Check sheet for the modelled part. Datum: model origin and axes. Units: mm. A direction names the side the tool comes from. Round coordinates to 2 decimals unless told otherwise and drop trailing zeros. Loops run counter-clockwise (first coordinate to the right, second up) from the corner with the lowest first, then second, coordinate; pieces in that order, holes last. Notation, with made-up numbers: (75, 52) -> (103, 52) arc R24 ccw to (103, 69) -> close; hole circle Ø10 at (29.25, 14.5). An arc over 180 degrees is marked (long way). Return JSON: item names as keys, results as strings.
from build123d import *

# Parameters (mm, degrees)
F0_W     = 76.597254
F0_H     = 76.218059
F1_DEPTH = 19.05
F2_R     = 25.573728
F3_DEPTH = 76.2
F4_W     = 76.946799
F4_H     = 75.848795
F5_DEPTH = 19.05
F8_D     = 12.7
F9_D     = 38.1


with BuildPart() as f1:
    # F0 (on Right) → F1 (new body)
    with BuildSketch(Plane.YZ):
        with Locations((-6.7307, 10.143448)):
            Rectangle(F0_W, F0_H)
    extrude(amount=F1_DEPTH)

    # F2 (on face) → F3 (join)
    with BuildSketch(Plane(origin=(0, 0, 0), x_dir=(0, -1, 0), z_dir=(-1, 0, 0))):
        with Locations((7.766344, 7.780468)):
            Circle(F2_R)
    extrude(amount=F3_DEPTH)

    # F4 (on face) → F5 (join)
    with BuildSketch(Plane(origin=(-76.2, 0, 0), x_dir=(0, -1, 0), z_dir=(-1, 0, 0))):
        with Locations((6.074561, 10.491825)):
            Rectangle(F4_W, F4_H)
    extrude(amount=F5_DEPTH)

    # F8 (through all)
    with Locations(Plane(origin=(-95.25, 0, 0), x_dir=(0, -1, 0), z_dir=(-1, 0, 0))):
        with Locations((-23.013473, -18.076902), (-24.134498, 37.203994), (35.561476, 38.338061), (35.561476, -18.081902)):
            Hole(F8_D / 2)

    # F9 (through all)
    with Locations(Plane(origin=(-95.25, 0, 0), x_dir=(0, -1, 0), z_dir=(-1, 0, 0))):
        with Locations((6.17749, 7.946953)):
            Hole(F9_D / 2)


solid = f1.part
Q1. Go/stop test with flat-tipped pins: pin 1 (6 mm diameter, centred on x = -67.5, z = 2, fed in from +Y); pin 2 (12 mm diameter, centred on x = -18.5, z = 18.5, fed in from +Y); pin 3 (5.5 mm diameter, centred on x = 8.5, y = -24, fed in from +Z). Record where each tip stops, or that it passes through.
Results list:
{"pin 1": "y = 17.66", "pin 2": "y = 17.37", "pin 3": "z = 48.25"}
Q2. Section check D-D (y = 20.5). Record the boundary of the cut face in (x, z), then the cut area to 3 significant figures.
Results list:
{"outline": "(-95.25, -27.43) -> (-76.2, -27.43) -> (-76.2, -23.91) -> (-95.25, -23.91) -> close; (-95.25, -12.25) -> (-76.2, -12.25) -> (-76.2, 32) -> (-95.25, 32) -> close; (-95.25, 42.41) -> (-76.2, 42.41) -> (-76.2, 48.42) -> (-95.25, 48.42) -> close; (0, -27.97) -> (19.05, -27.97) -> (19.05, -23.91) -> (0, -23.91) -> close; (0, -12.25) -> (19.05, -12.25) -> (19.05, 32) -> (0, 32) -> close; (0, 42.41) -> (19.05, 42.41) -> (19.05, 48.25) -> (0, 48.25) -> close", "area": "2,060 mm^2"}
Q3. Material ranges on line 1 (Z direction, x = -33, y = -7); line 2 (Y direction, x = -51, z = 7.5); line 3 (X direction, y = 1, z = -16.5), recorded low to high.
Results list:
{"line 1": "-17.78 to -11.09, 26.98 to 33.34", "line 2": "-33.34 to -25.22, 12.87 to 17.81", "line 3": "-95.25 to -76.2, 0 to 19.05"}
Q4. Tool access check on faces 4 (the flat face through (9, -7, 48.252)), 5 (the flat face through (-86, -44.548, 10)), 6 (the flat face through (-76.2, 12, 28)). Record the directions out of +Z, -Z, +X, -X, +Y, -Y that give a thin tool (end or side, any length) a straight path to the whole face; none if there is none.
Results list:
{"face 4": "+Z, +X, +Y, -Y", "face 5": "+Z, -Z, -X, -Y", "face 6": "none"}
Q5. Section check B-B (y = -9). Record the boundary of the cut face in (x, z).
Results list:
{"outline": "(-95.25, -27.43) -> (-76.2, -27.43) -> (-76.2, -17.76) -> (0, -17.76) -> (0, -27.97) -> (19.05, -27.97) -> (19.05, -10.89) -> (-95.25, -10.89) -> close; (-95.25, 26.79) -> (19.05, 26.79) -> (19.05, 48.25) -> (0, 48.25) -> (0, 33.32) -> (-76.2, 33.32) -> (-76.2, 48.42) -> (-95.25, 48.42) -> close"}
Q6. Section check C-C (z = 18). Record the boundary of the cut face in (x, y).
Results list:
{"outline": "(-95.25, -44.55) -> (-76.2, -44.55) -> (-76.2, -31.21) -> (0, -31.21) -> (0, -45.03) -> (19.05, -45.03) -> (19.05, -22.36) -> (-95.25, -22.36) -> close; (-95.25, 10) -> (19.05, 10) -> (19.05, 31.57) -> (0, 31.57) -> (0, 15.68) -> (-76.2, 15.68) -> (-76.2, 32.4) -> (-95.25, 32.4) -> close"}
Q7. Section check A-A (z = -20.5). Record the boundary of the cut face in (x, y), then the cut area to 3 significant figures.
Results list:
{"outline": "(-95.25, -44.55) -> (-76.2, -44.55) -> (-76.2, -41.43) -> (-95.25, -41.43) -> close; (-95.25, -29.69) -> (-76.2, -29.69) -> (-76.2, 17.14) -> (-95.25, 17.14) -> close; (-95.25, 28.88) -> (-76.2, 28.88) -> (-76.2, 32.4) -> (-95.25, 32.4) -> close; (0, -45.03) -> (19.05, -45.03) -> (19.05, -41.43) -> (0, -41.43) -> close; (0, -29.69) -> (19.05, -29.69) -> (19.05, 17.14) -> (0, 17.14) -> close; (0, 28.88) -> (19.05, 28.88) -> (19.05, 31.57) -> (0, 31.57) -> close", "area": "2,030 mm^2"}
Q8. Draft check along Y on faces 1 (the flat face through (9, 31.568, 10)), 2 (the cylindrical face through (-85.592, -32.631, 32.705)), 3 (the flat face through (19.05, -7, 28)). Enter one of: released by +Y, released by -Y, zero draft, split by the parting line, or undercut.
Results list:
{"face 1": "released by +Y", "face 2": "undercut", "face 3": "zero draft"}
